For this review, take the finished solid that the model builds, in its own axes (mm). Face numbers are marked on the shaded views. A direction names the side the tool comes from. Coordinates: 2 decimals unless noted, no trailing zeros. Loops run counter-clockwise (first coordinate to the right, second up) from the corner with the lowest first, then second, coordinate; pieces in that order, holes last. Notation, with made-up numbers: (-22, 48) -> (-2, 48) arc R18 ccw to (-2, 60) -> close; hole circle Ø11 at (44.5, 8). An arc over 180 degrees is marked (long way). One line per item, written item: value.
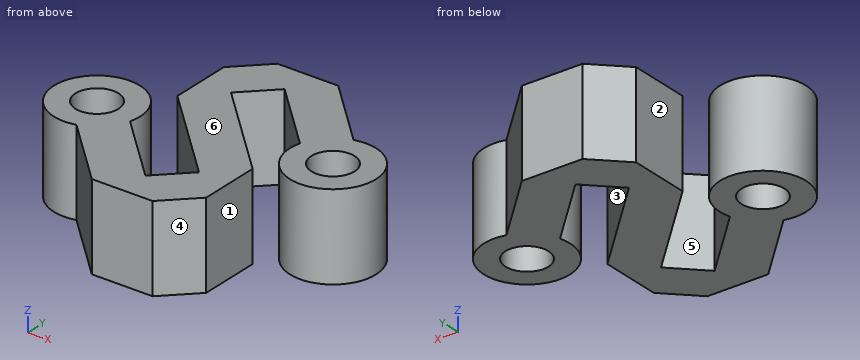
Autodesk Inventor part; units mm, degrees
ref_plane "YZ Plane" through (0, 0, 0) normal (1, 0, 0) x (0, 1, 0)
ref_plane "XZ Plane" through (0, 0, 0) normal (0, 1, 0) x (-1, 0, 0)
ref_plane "XY Plane" through (0, 0, 0) normal (0, 0, 1) x (1, 0, 0)
sketch "Sketch1" plane through (0, 0, 0) normal (0, 0, 1) x (1, 0, 0)
  circle A0 centre (0, 0) radius 2.5
  circle A1 centre (0, 0) radius 5
  line L0 (-1.7678, -1.7678) -> (-12.3744, 8.8388)
  line L1 (-12.3744, 8.8388) -> (-15.9099, 5.3033)
  line L2 (-15.9099, 5.3033) -> (-5.3033, -5.3033)
  line L3 (-5.3033, -5.3033) -> (-5.3033, -12.3744)
  line L4 (-5.3033, -12.3744) -> (-8.8388, -15.9099)
  line L5 (-15.9099, -15.9099) -> (-26.5165, -5.3033)
  line L6 (1.7678, 1.7678) -> (-8.8388, 12.3744)
  line L7 (-15.9099, 12.3744) -> (-19.4454, 8.8388)
  line L8 (-19.4454, 8.8388) -> (-19.4454, 1.7678)
  line L9 (-19.4454, 1.7678) -> (-8.8388, -8.8388)
  line L10 (-8.8388, -8.8388) -> (-12.3744, -12.3744)
  line L11 (-12.3744, -12.3744) -> (-22.981, -1.7678)
  line L12 (-22.981, -1.7678) -> (-26.5165, -5.3033)
  line L13 (-1.7678, -1.7678) -> (1.7678, 1.7678)
  circle A2 centre (-24.7487, -3.5355) radius 2.5
  circle A3 centre (-24.7487, -3.5355) radius 5
  line L14 (-15.9099, 12.3744) -> (-8.8388, 12.3744)
  line L15 (-15.9099, -15.9099) -> (-8.8388, -15.9099)
  dimension "d0" = 5
  dimension "d1" = 10
  dimension "d3" = 90
  dimension "d6" = 135
  dimension "d7" = 135
  dimension "d8" = 90
  dimension "d9" = 5
  dimension "d12" = 10
  dimension "d13" = 15
  dimension "d14" = 15
  dimension "d31" = 7.0711
  dimension "d32" = 15
  dimension "d33" = 7.0711
  dimension "d34" = 15
  dimension "d35" = 7.0711
  dimension "d36" = 7.0711
  dimension "d37" = 5
  dimension "d38" = 90
  dimension "d39" = 135
  dimension "d40" = 5
  dimension "d41" = 5
extrude "Extrusion4" add sketch "Sketch1" along normal blind 10 contours A0 L6 A1 L0 | A0 L0 A1 L6 | A1 L0 L1 L2 L3 L4 L15 L5 A3 L11 L10 L9 L8 L7 L14 L6 | A3 L5 A2 L11 | L11 A2 L5 A3 | A2 L12 picked at (-25.0062, -4.328)
sketch "Sketch3" plane through (0, 0, 10) normal (0, 0, 1) x (1, 0, 0)
  line L0 (-1.2941, 4.8296) -> (-8.8388, 12.3744)
  line L1 (-8.8388, 12.3744) -> (-15.9099, 12.3744)
  line L2 (-15.9099, 12.3744) -> (-19.4454, 8.8388)
  line L3 (-19.4454, 8.8388) -> (-19.4454, 1.7678)
  line L4 (-19.4454, 1.7678) -> (-8.8388, -8.8388)
  line L5 (-8.8388, -8.8388) -> (-12.3744, -12.3744)
  line L6 (-12.3744, -12.3744) -> (-19.9191, -4.8296)
  arc A0 (-19.9191, -4.8296) -> (-23.4546, -8.3652) centre (-24.7487, -3.5355) ccw
  line L7 (-23.4546, -8.3652) -> (-15.9099, -15.9099)
  line L8 (-15.9099, -15.9099) -> (-8.8388, -15.9099)
  line L9 (-8.8388, -15.9099) -> (-5.3033, -12.3744)
  line L10 (-5.3033, -12.3744) -> (-5.3033, -5.3033)
  line L11 (-5.3033, -5.3033) -> (-15.9099, 5.3033)
  line L12 (-15.9099, 5.3033) -> (-12.3744, 8.8388)
  line L13 (-12.3744, 8.8388) -> (-4.8296, 1.2941)
  arc A1 (-4.8296, 1.2941) -> (-1.2941, 4.8296) centre (0, 0) ccw
  line L14 (-26.5165, -5.3033) -> (-22.981, -1.7678)
  arc A2 (-22.981, -1.7678) -> (-26.5165, -5.3033) centre (-24.7487, -3.5355) ccw
  circle A3 centre (0, 0) radius 2.5
  circle A4 centre (-24.7487, -3.5355) radius 2.5
extrude "Extrusion5" cut sketch "Sketch3" against normal blind 10 contours L14 A4
equation "\"d1\" = 2 * d0"
equation "\"d9\" = d0"
equation "\"d12\" = d1"
equation "\"d13\" = 3 * d0"
equation "\"d14\" = d13"
properties part number "Sawaiz Logo Ribbon"
1. Take a section at D-D, the plane y = 0. Give the boundary of the cut face in (x, z), and give its area (3 significant figures).
Return value:
outline: (-28.28, 0) -> (-21.21, 0) -> (-21.21, 10) -> (-28.28, 10) -> close; (-17.68, 0) -> (-10.61, 0) -> (-10.61, 10) -> (-17.68, 10) -> close; (-5, 0) -> (-2.5, 0) -> (-2.5, 10) -> (-5, 10) -> close; (2.5, 0) -> (5, 0) -> (5, 10) -> (2.5, 10) -> close
area: 191 mm2
2. Take a section at A-A, the plane x = 0. Give the boundary of the cut face in (y, z).
Return value:
outline: (-5, 0) -> (-2.5, 0) -> (-2.5, 10) -> (-5, 10) -> close; (2.5, 0) -> (5, 0) -> (5, 10) -> (2.5, 10) -> close
3. Insertion check: pin 1 Ø5.5 at (y, z) = (-9.5, 4.5) entering from +X; pin 2 Ø5 at (x, z) = (-20.5, 4.5) entering from -Y; pin 3 Ø3.5 at (y, z) = (7, 3) entering from -X. Each pin has a flat end and moves straight along its axis. Give the tip position at first contact, or say it passes through.
Return value:
pin 1: stops at x = -5.3
pin 2: stops at y = -13.82
pin 3: stops at x = -19.45
4. For the marked faces 1, 2 and 3, list the 3-axis set-ups (+Z, -Z, +X, -X, +Y, -Y) from which the entire face can be reached by the end or side of a thin tool; tool diameter is ignored.
Return value:
face 1: +Z, -Z, +X, -Y
face 2: +Z, -Z, -X, +Y
face 3: +Z, -Z
5. Take a section at C-C, the plane z = 7.5. Give the boundary of the cut face in (x, y), and give its area (3 significant figures).
Return value:
outline: (-23.45, -8.37) -> (-15.91, -15.91) -> (-8.84, -15.91) -> (-5.3, -12.37) -> (-5.3, -5.3) -> (-15.91, 5.3) -> (-12.37, 8.84) -> (-4.83, 1.29) arc R5 ccw (long way) to (-1.29, 4.83) -> (-8.84, 12.37) -> (-15.91, 12.37) -> (-19.45, 8.84) -> (-19.45, 1.77) -> (-8.84, -8.84) -> (-12.37, -12.37) -> (-19.92, -4.83) arc R5 ccw (long way) to start; hole circle Ø5 at (-24.75, -3.54); hole circle Ø5 at (0, 0)
area: 395 mm2
6. Take a section at B-B, the plane x = -15.5. Give the boundary of the cut face in (y, z), and give its area (3 significant figures).
Return value:
outline: (-15.91, 0) -> (-9.25, 0) -> (-9.25, 10) -> (-15.91, 10) -> close; (-2.18, 0) -> (4.89, 0) -> (4.89, 10) -> (-2.18, 10) -> close; (5.71, 0) -> (12.37, 0) -> (12.37, 10) -> (5.71, 10) -> close
area: 204 mm2
7. To check wall thickness, follow probe 1 along Y at (x, z) = (-10.5, 6.5); probe 2 along Y at (x, z) = (0, 6.25); probe 3 along X at (y, z) = (0, 4.25). State the ranges of each line that lie inside material, in increasing order. Write a range as from..to.
Return value:
probe 1: y = -15.91..-10.5, -7.18..-0.11, 6.96..12.37
probe 2: y = -5..-2.5, 2.5..5
probe 3: x = -28.28..-21.21, -17.68..-10.61, -5..-2.5, 2.5..5
8. The part is to be moulded in two halves that separate along Y. For the marked faces 4, 5 and 6, say which applies: pulls with the +Y half, pulls with the -Y half, needs draft (parallel to the pull), parting line crosses it, or undercut.
Return value:
face 4: pulls with the -Y half
face 5: undercut
face 6: needs draft
